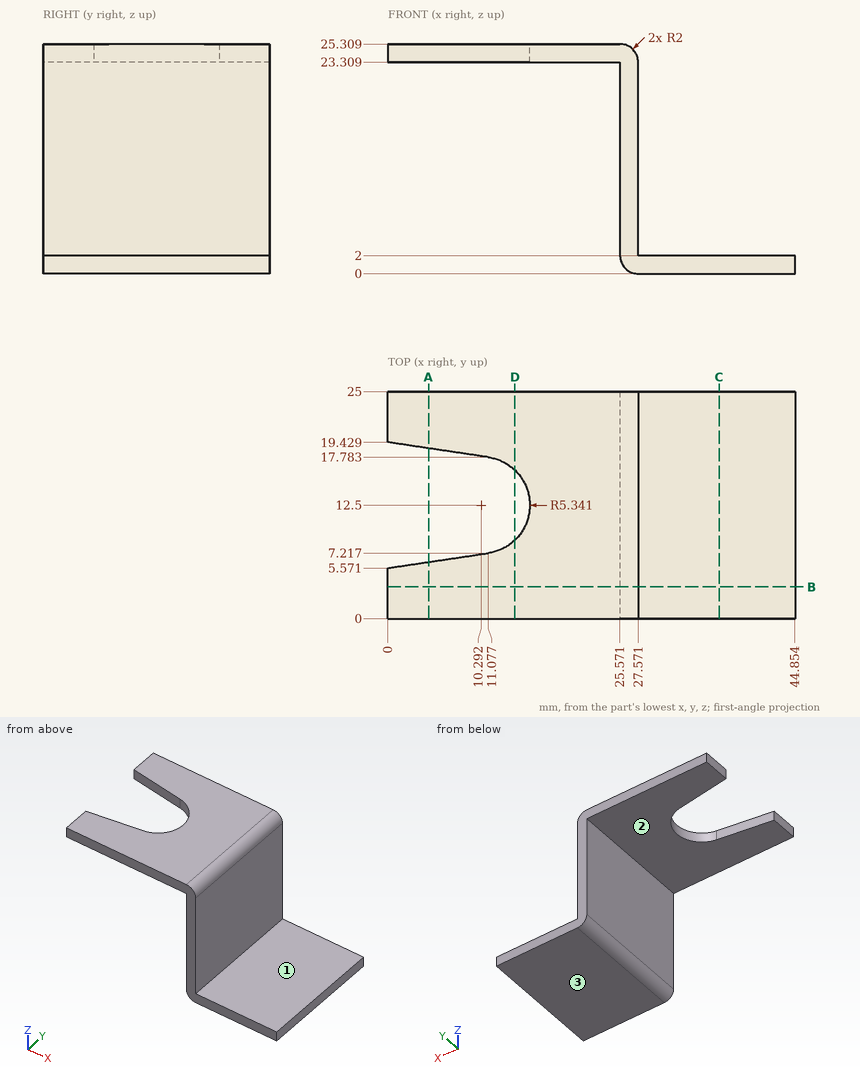
Geometry: see drawing. Coordinates: mm, zero at the bounding-box minimum. A direction names the side the tool comes from. Coordinates: 2 decimals unless noted, no trailing zeros. Loops run counter-clockwise (first coordinate to the right, second up) from the corner with the lowest first, then second, coordinate; pieces in that order, holes last.
(1) Material intervals for probe 1 along X at (y, z) = (5.5, 12.5); probe 2 along Z at (x, y) = (38, 13.25); probe 3 along Z at (x, y) = (13, 21), sorted ascending.
(2) Set-up query: the marked faces 1, 2 and 3. Return all of +Z, -Z, +X, -X, +Y, -Y with unobstructed straight access to the full face (end or side cutting, diameter ignored); none if empty.
(3) Section A-A on x = 4.5. Return the cut outline in (y, z).
(4) Section C-C on x = 36.5. Return the cut outline in (y, z).
(5) Section B-B on y = 3.5. Return the cut outline in (x, z) (1 decimal).
(6) First-contact query: pin 1 Ø12 at (x, z) = (36.5, 21) entering from +Y; pin 2 Ø8.5 at (x, y) = (37.5, 7.5) entering from +Z; pin 3 Ø6.5 at (y, z) = (16, 14) entering from +X; pin 4 Ø10.5 at (y, z) = (12.5, 13) entering from -X. Flat tips, straight axial feed; report the tip coordinate or a pass-through.
(7) Section D-D on x = 14. Return the cut outline in (y, z).
Data:
1. probe 1: x = 25.57 to 27.57
1. probe 2: z = 0 to 2
1. probe 3: z = 23.31 to 25.31
2. face 1: +Z, +X, +Y, -Y
2. face 2: -Z, -X, +Y, -Y
2. face 3: -Z, +X, -X, +Y, -Y
3. outline: (0, 23.31) - (6.24, 23.31) - (6.24, 25.31) - (0, 25.31) - close; (18.76, 23.31) - (25, 23.31) - (25, 25.31) - (18.76, 25.31) - close
4. outline: (0, 0) - (25, 0) - (25, 2) - (0, 2) - close
5. outline: (0, 23.3) - (25.6, 23.3) - (25.6, 2) arc R2 ccw to (27.6, 0) - (44.9, 0) - (44.9, 2) - (27.6, 2) - (27.6, 23.3) arc R2 ccw to (25.6, 25.3) - (0, 25.3) - close
6. pin 1: passes through
6. pin 2: stops at z = 2
6. pin 3: stops at x = 27.57
6. pin 4: stops at x = 25.57
7. outline: (0, 23.31) - (8.66, 23.31) - (8.66, 25.31) - (0, 25.31) - close; (16.34, 23.31) - (25, 23.31) - (25, 25.31) - (16.34, 25.31) - close
